from build123d import *

# Parameters (mm, degrees)
CROQUIS1_W              = 4.7625
CROQUIS1_H              = 42.333333333
SALIENTE_EXTRUIR1_DEPTH = 25.4
CROQUIS2_R              = 3.96875
CORTAR_EXTRUIR1_DEPTH   = 25.4


with BuildPart() as part:
    # Croquis1 → Saliente-Extruir1 (new body)
    with BuildSketch(Plane(origin=(0, 0, 0), x_dir=(1, 0, 0), z_dir=(0, 1, 0))):
        with Locations((604.572916667, 432.985333334)):
            Rectangle(CROQUIS1_W, CROQUIS1_H)
    extrude(amount=SALIENTE_EXTRUIR1_DEPTH)

    # Croquis2 → Cortar-Extruir1 (cut)
    with BuildSketch(Plane(origin=(606.954166667, 0, 0), x_dir=(0, 0, -1), z_dir=(1, 0, 0))):
        with BuildLine():
            ThreePointArc((426.635333333, 19.05), (428.495205273, 23.540128061), (432.985333333, 25.4))
            Line((432.985333333, 25.4), (411.818666667, 25.4))
            Line((411.818666667, 25.4), (411.818666667, 0))
            Line((411.818666667, 0), (413.935333333, 0))
            Line((413.935333333, 0), (413.935333333, 2.12))
            ThreePointArc((413.935333333, 2.12), (423.10744442, 8.467999953), (426.635333333, 19.05))
        make_face()
        with BuildLine():
            ThreePointArc((432.985333333, 25.4), (437.475461394, 23.540128061), (439.335333333, 19.05))
            Line((439.335333333, 19.05), (439.335333333, 0))
            Line((439.335333333, 0), (454.152, 0))
            Line((454.152, 0), (454.152, 25.4))
            Line((454.152, 25.4), (432.985333333, 25.4))
        make_face()
        with Locations((432.985333333, 19.05)):
            Circle(CROQUIS2_R)
    extrude(amount=-CORTAR_EXTRUIR1_DEPTH, mode=Mode.SUBTRACT)


solid = part.part
Geometry check sheet. Reference: the model listing, model coordinates, mm. Round coordinates to 2 decimals unless told otherwise and drop trailing zeros. Order: outer loops, then holes, each group sorted by start corner. A loop starts at its lowest first (then second) coordinate and runs counter-clockwise, first axis right, second up. Notation, with made-up numbers: M 55,29 L 96,29 A10 ccw 96,38 Z; hole C -19,61.5 d10. An arc over 180 degrees is marked long. Write each question's results on one line, items separated by ' | '. Start each with the question number.
1. Material ranges on L1, parallel to Y at x = 605.9, z = -433.75; L2, parallel to Y at x = 606.15, z = -436.25; L3, parallel to Z at x = 605.9, y = 18.5, recorded low to high. Write a range as from..to.
2. Draft check along Y on faces 1 (the face through (604.61, 20.24, -436.77)), 2 (the face through (602.192, 10, -429)), 3 (the face through (605, 0, -427)). Enter one of: pulls with the +Y half, pulls with the -Y half, needs draft (parallel to the pull), parting line crosses it, or undercut.
3. Cross-section at A-A on z = -435.5. Record the boundary of the cut face in (x, y).
4. Go/stop test with a flat-tipped pin: P1, Ø1.5, axis at y = 18, z = -435.5, coming from the +X side. Record where the tip stops, or that it passes through.
5. Cross-section at C-C on z = -432.5. Record the boundary of the cut face in (x, y), plus the area to 3 significant figures.
6. Cross-section at D-D on y = 23.75. Record the boundary of the cut face in (x, z).
7. Cross-section at B-B on x = 604.65. Record the boundary of the cut face in (y, z).
Resolved:
1) L1: 0..15.16, 22.94..25.35 | L2: 0..16.79, 21.31..24.5 | L3: -439.34..-436.92, -429.05..-426.63
2) face 1: undercut | face 2: needs draft | face 3: pulls with the -Y half
3) outline: M 602.19,0 L 606.95,0 L 606.95,15.98 L 602.19,15.98 Z; M 602.19,22.12 L 606.95,22.12 L 606.95,24.88 L 602.19,24.88 Z
4) P1: through
5) outline: M 602.19,0 L 606.95,0 L 606.95,15.11 L 602.19,15.11 Z; M 602.19,22.99 L 606.95,22.99 L 606.95,25.38 L 602.19,25.38 Z | area: 83.4 mm2
6) outline: M 602.19,-437.26 L 606.95,-437.26 L 606.95,-428.72 L 602.19,-428.72 Z
7) outline: M 0,-439.34 L 19.05,-439.34 A6.35 ccw 19.05,-426.64 A17.63 cw 2.12,-413.94 L 0,-413.94 Z; hole C 19.05,-432.99 d7.94
